Here's the drawing with two shaded views (mm, measured from the low corner). I have some questions. Give positions to 0.01 mm unless a question says otherwise; leave off trailing zeros. Write each loop counter-clockwise with the first axis right and the second up, starting at its lowest first coordinate (ties: lowest second). Pieces come first, ordered by that corner, then holes.
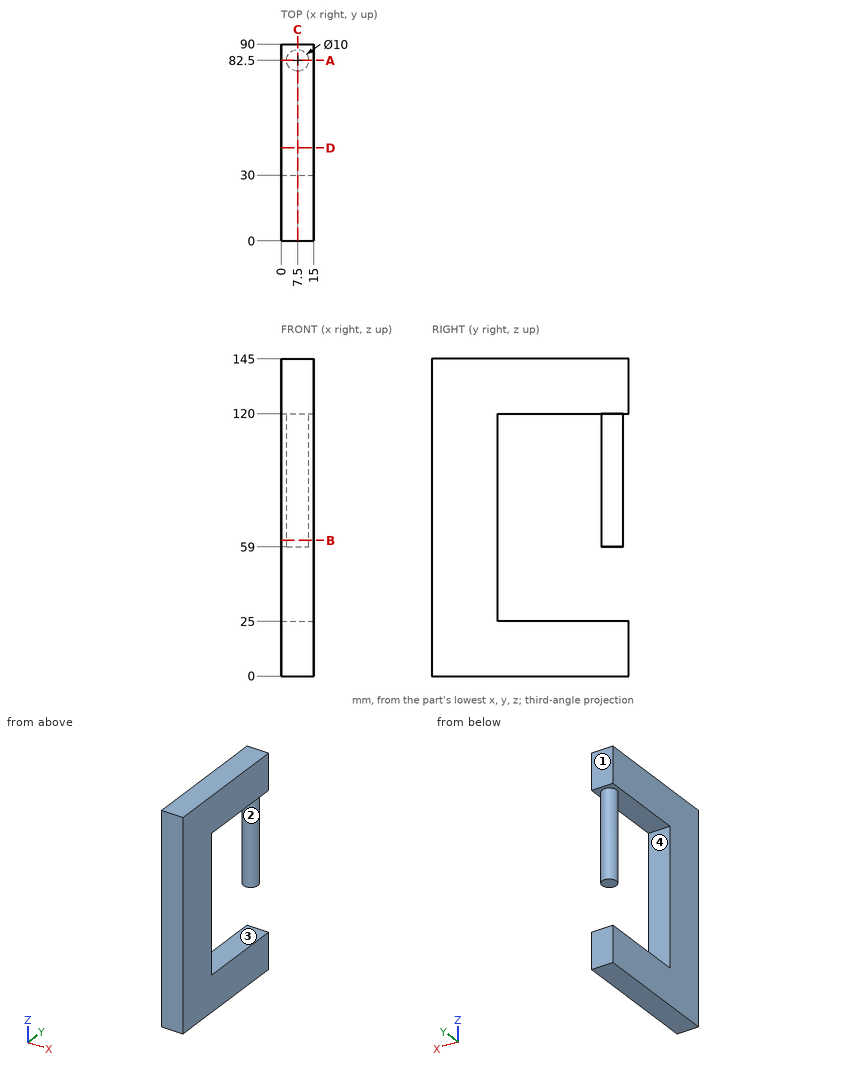
1) If we mould it in two halves opening along Y, with no side actions, what happens to the marked faces 1, 2, 3 and 4? For each: +Y half, -Y half, draft (parallel to the pull), parting line (faces both ways), or undercut.
Values follow:
face 1: +Y half
face 2: undercut
face 3: draft
face 4: undercut
2) Suppose I cut it at A-A on y = 82.5. Write out the boundary of the cut face in (x, z).
Values follow:
outline: (0, 0) - (15, 0) - (15, 25) - (0, 25) - close; (0, 120) - (2.5, 120) - (2.5, 59) - (12.5, 59) - (12.5, 120) - (15, 120) - (15, 145) - (0, 145) - close
3) Suppose I cut it at C-C on x = 7.5. Write out the boundary of the cut face in (y, z).
Values follow:
outline: (0, 0) - (90, 0) - (90, 25) - (30, 25) - (30, 120) - (77.5, 120) - (77.5, 59) - (87.5, 59) - (87.5, 120) - (90, 120) - (90, 145) - (0, 145) - close
4) Suppose I cut it at D-D on y = 42.5. Write out the boundary of the cut face in (x, z).
Values follow:
outline: (0, 0) - (15, 0) - (15, 25) - (0, 25) - close; (0, 120) - (15, 120) - (15, 145) - (0, 145) - close
5) Suppose I cut it at B-B on z = 62. Write out the boundary of the cut face in (x, y), plus the area to 3 significant figures.
Values follow:
outline: (0, 0) - (15, 0) - (15, 30) - (0, 30) - close; circle Ø10 at (7.5, 82.5)
area: 529 mm2
6) Please list where these lines run through material, in increasing order: L1, parallel to Y at x = 8, z = 108; L2, parallel to Z at x = 2, y = 85.5; L3, parallel to Z at x = 9.25, y = 79.
Values follow:
L1: y = 0 to 30, 77.53 to 87.47
L2: z = 0 to 25, 120 to 145
L3: z = 0 to 25, 59 to 145
7) For pin 1 Ø4.5 at (x, z) = (7, 81) entering from +Y, with a flat end and sliding along its axis, tell me the tip position at first contact or that it passes through.
Values follow:
pin 1: stops at y = 87.5
